```python
from build123d import *

# Parameters (mm, degrees)
F0_W      = 15
F0_H      = 8
F1_DEPTH  = 15
F1_TAPER  = 3
F2_R      = 2.5
F3_DEPTH  = 5
F4_R      = 1
F5_R      = 1.5
F6_DEPTH  = 3
F7_R      = 1.5
F6_FACE_R = 1.5
F8_DEPTH  = 3


with BuildPart() as f1:
    # F0 (on Top) → F1 (new body)
    with BuildSketch(Plane.XY):
        Rectangle(F0_W, F0_H)
    extrude(amount=F1_DEPTH, taper=F1_TAPER)

    # F2 (on face) → F3 (join)
    with BuildSketch(Plane.XY.offset(15)):
        Circle(F2_R)
    extrude(amount=F3_DEPTH)

    # F4
    f4_edges = [f1.edges().sort_by_distance(p)[0] for p in [
        (0, 3.213883, 15),
        (-7.106942, 3.606942, 7.5),
        (7.106942, 3.606942, 7.5),
        (-7.106942, -3.606942, 7.5),
        (-6.713883, 0, 15),
        (0, -3.213883, 15),
        (7.106942, -3.606942, 7.5),
        (6.713883, 0, 15),
    ]]
    fillet(f4_edges, radius=F4_R)

    # F5 (on face) → F6 (cut)
    with BuildSketch(Plane(origin=(-7.4794571076, 0, 0.3919817373), x_dir=(0, -1, 0), z_dir=(-0.9986295348, 0, 0.0523359562))):
        with Locations((0, 10.6777304862)):
            Circle(F5_R)
    extrude(amount=-F6_DEPTH, mode=Mode.SUBTRACT)

    # F7 (on face) + F6_face (on face) → F8 (cut)
    with BuildSketch(Plane(origin=(7.4794571076, 0, 0.3919817373), x_dir=(0, 1, 0), z_dir=(0.9986295348, 0, 0.0523359562))):
        with Locations((0, 10.6777304862)):
            Circle(F7_R)
    with BuildSketch(Plane(origin=(-3.9247392679, 0, 10.8980708962), x_dir=(0, -1, 0), z_dir=(-0.9986295348, 0, 0.0523359562))):
        Circle(F6_FACE_R)
    extrude(amount=-F8_DEPTH, dir=(0.9986295348, 0, 0.0523359562), mode=Mode.SUBTRACT)


solid = f1.part
```
Check sheet for the modelled part. Datum: model origin and axes. Units: mm. A direction names the side the tool comes from. Give positions to 0.01 mm unless a question says otherwise; leave off trailing zeros. Write each loop counter-clockwise with the first axis right and the second up, starting at its lowest first coordinate (ties: lowest second). Pieces come first, ordered by that corner, then holes. Notation, with made-up numbers: (30, 15.25) - (46, 15.25) arc R30 ccw to (46, 46.25) - close; hole circle Ø4 at (13.25, 13.5). An arc over 180 degrees is marked (long way). Answer as a JSON object with one key per item and string values. Group by question number.
1) Depth check by flat-ended pin: P1, Ø4, axis at x = 4.5, y = 1.5, coming from the +Z side; P2, Ø6, axis at x = -4.5, z = 2.5, coming from the -Y side; P3, Ø4, axis at y = -2.5, z = 14.5, coming from the +X side; P4, Ø8, axis at x = 2.5, z = 11, coming from the -Y side. Enter the tip coordinate at first touch or a pass-through.
2) Access from +Z, -Z, +X, -X, +Y, -Y to the whole of each face (thin tool, end or side, straight path). Record for faces 5 (the face through (-0.54, -2.44, 17.46)), 6 (the face through (3.44, -2.96, 14.72)), 7 (the face through (-3.44, 2.96, 14.72)), 8 (the face through (-6.46, -0.03, 14.72)).
3) Sectioned sample at A-A (x = -3.5). Record the cut outline in (y, z), then the cut area to 3 significant figures.
4) Thickness scan on probe 1 along X at (y, z) = (1.5, 9.5); probe 2 along Z at (x, y) = (-2.5, -1.5); probe 3 along X at (y, z) = (0, 15.75). Record the ranges inside material, lowest first. Write a range as from..to.
5) Release check for a two-part mould opening along X. For faces 1 (the face through (-6.84, -3.33, 7.13)), 2 (the face through (0, 0, 20)), 3 (the face through (5.513, 0.692, 9.649)), 4 (the face through (6.84, 3.33, 7.13)) record: pulls with the +X half, pulls with the -X half, needs draft (parallel to the pull), parting line crosses it, or undercut.
Geometry results:
{
 "1": {"P1": "stops at z = 15", "P2": "stops at y = -4", "P3": "stops at x = 6.84", "P4": "stops at y = -3.63"},
 "2": {"face 5": "+Z", "face 6": "+Z, +X, -Y", "face 7": "+Z, -X, +Y", "face 8": "+Z, -X, +Y, -Y"},
 "3": {"outline": "(-4, 0) - (4, 0) - (3.26, 14.05) arc R1 ccw to (2.26, 15) - (-2.26, 15) arc R1 ccw to (-3.26, 14.05) - close", "area": "108 mm^2"},
 "4": {"probe 1": "x = -7..7", "probe 2": "z = 0..15", "probe 3": "x = -2.5..2.5"},
 "5": {"face 1": "pulls with the -X half", "face 2": "needs draft", "face 3": "undercut", "face 4": "pulls with the +X half"}
}
